from build123d import *

# Parameters (mm, degrees)
SKETCH_1_R                     = 17
EXTRUDE_1_DEPTH                = 3
SKETCH_2_R                     = 17
SKETCH_2_R_2                   = 15
EXTRUDE_2_DEPTH                = 40
SKETCH_3_R                     = 5
CUT_EXTRUDE_1_DEPTH            = 4
SKETCH_4_R                     = 17
EXTRUDE_3_DEPTH                = 7
SKETCH_5_W                     = 20.2
SKETCH_5_H                     = 20.2
EXTRUDE_4_DEPTH                = 30
HOLE_WIZARD_M5_2_D             = 5.5
HOLE_WIZARD_M5_2_CSINK_D       = 5.55
HOLE_WIZARD_M5_2_CSINK_ANGLE   = 90
HOLE_WIZARD_M2_5_2_D           = 2.9
HOLE_WIZARD_M2_5_2_DEPTH       = 3
HOLE_WIZARD_M2_5_2_CSINK_D     = 2.95
HOLE_WIZARD_M2_5_2_CSINK_ANGLE = 90
SKETCH_12_W                    = 47.187362465
SKETCH_12_H                    = 89.366632215
CUT_EXTRUDE_2_DEPTH            = 18


with BuildPart() as part:
    # 草图1 → 凸台-拉伸1 (new body)
    with BuildSketch(Plane.XY):
        Circle(SKETCH_1_R)
    extrude(amount=EXTRUDE_1_DEPTH)

    # 草图2 → 凸台-拉伸2 (add)
    with BuildSketch(Plane.XY.offset(3)):
        Circle(SKETCH_2_R)
        Circle(SKETCH_2_R_2, mode=Mode.SUBTRACT)
    extrude(amount=EXTRUDE_2_DEPTH)

    # 草图3 → 切除-拉伸1 (cut, through all)
    with BuildSketch(Plane.XY.offset(3)):
        Circle(SKETCH_3_R)
    extrude(amount=-CUT_EXTRUDE_1_DEPTH, mode=Mode.SUBTRACT)

    # 草图4 → 凸台-拉伸3 (add)
    with BuildSketch(Plane.XY.offset(43)):
        Circle(SKETCH_4_R)
        Polygon((-4.443145751, 10.1), (4.443145751, 10.1), (10.1, 4.443145751), (10.1, -4.443145751), (4.443145751, -10.1), (-4.443145751, -10.1), (-10.1, -4.443145751), (-10.1, 4.443145751), align=None, mode=Mode.SUBTRACT)
    extrude(amount=EXTRUDE_3_DEPTH)

    # 草图5 → 凸台-拉伸4 (add)
    with BuildSketch(Plane.XY.offset(50)):
        with BuildLine():
            Line((9.49684158, 14.1), (-9.49684158, 14.1))
            ThreePointArc((-9.49684158, 14.1), (-12.02081528, 12.02081528), (-14.1, 9.49684158))
            Line((-14.1, 9.49684158), (-14.1, -9.496842588))
            ThreePointArc((-14.1, -9.496842588), (-12.020815678, -12.020815678), (-9.496842588, -14.1))
            Line((-9.496842588, -14.1), (9.49684158, -14.1))
            ThreePointArc((9.49684158, -14.1), (12.02081528, -12.02081528), (14.1, -9.49684158))
            Line((14.1, -9.49684158), (14.1, 9.49684158))
            ThreePointArc((14.1, 9.49684158), (12.02081528, 12.02081528), (9.49684158, 14.1))
        make_face()
        Rectangle(SKETCH_5_W, SKETCH_5_H, mode=Mode.SUBTRACT)
    extrude(amount=EXTRUDE_4_DEPTH)

    # M5 间隙孔2 (through all)
    with Locations(Plane(origin=(0, 14.1, 0), x_dir=(1, 0, 0), z_dir=(0, 1, 0))):
        with Locations((0, -56), (0, -71)):
            CounterSinkHole(HOLE_WIZARD_M5_2_D / 2, HOLE_WIZARD_M5_2_CSINK_D / 2, counter_sink_angle=HOLE_WIZARD_M5_2_CSINK_ANGLE)

    # M2.5 间隙孔2
    with Locations(Plane.XY.offset(3)):
        with Locations((11, 0), (7.778174593, -7.778174593), (0, -11), (-7.778174593, -7.778174593), (-11, 0), (-7.778174593, 7.778174593), (0, 11), (7.778174593, 7.778174593)):
            CounterSinkHole(HOLE_WIZARD_M2_5_2_D / 2, HOLE_WIZARD_M2_5_2_CSINK_D / 2, depth=HOLE_WIZARD_M2_5_2_DEPTH, counter_sink_angle=HOLE_WIZARD_M2_5_2_CSINK_ANGLE)

    # 草图12 → 切除-拉伸2 (cut)
    with BuildSketch(Plane(origin=(0, 0, 0), x_dir=(1, 0, 0), z_dir=(0, 1, 0))):
        with Locations((-0.779036645, -41.61129095)):
            Rectangle(SKETCH_12_W, SKETCH_12_H)
    extrude(amount=-CUT_EXTRUDE_2_DEPTH, mode=Mode.SUBTRACT)


solid = part.part
Read the model definition and answer for the solid it produces. Units are mm, in the model's axes. A direction names the side the tool comes from. Round coordinates to 2 decimals unless told otherwise and drop trailing zeros. Write each loop counter-clockwise with the first axis right and the second up, starting at its lowest first coordinate (ties: lowest second). Pieces come first, ordered by that corner, then holes.
1. The part is cut by section C-C, the plane y = 11. Determine the outline of the cut face in (x, z) (3 decimals).
2. The part is cut by section A-A, the plane x = 0. Determine the outline of the cut face in (y, z) (3 decimals), then the cut area to 3 significant figures.
3. Straight lines are drawn through the part: L1, parallel to Z at x = 0, y = 11.6; L2, parallel to X at y = 5.75, z = 77; L3, parallel to Z at x = 0, y = 12.7. For each, find the intervals that lie inside material, in ascending order.
4. Determine the mould class of faces 6 (the face through (-14, 0, 48)), 7 (the face through (0, 11, 43)), 8 (the face through (-0.2, 10.3, 80)) for opening direction Z: pulls with the +Z half, pulls with the -Z half, needs draft (parallel to the pull), parting line crosses it, or undercut.
5. Given pin 1 Ø12 at (x, z) = (10, 24) entering from +Y; pin 2 Ø4.5 at (x, y) = (-2.5, 4) entering from +Z; pin 3 Ø2.5 at (x, y) = (-7.78, 7.78) entering from -Z; pin 4 Ø3.5 at (x, z) = (0, 71) entering from +Y, each flat-ended and moving along its own axis, determine where each tip first touches the part or whether it passes through.
6. The part is cut by section B-B, the plane z = 56. Determine the outline of the cut face in (x, y) (3 decimals), then the cut area to 3 significant figures.
7. Which of the six approach directions +Z, -Z, +X, -X, +Y, -Y give full straight-line access (tool end or side, diameter ignored) to faces 1 (the face through (14.1, 5, 65)), 2 (the face through (-14.1, 5, 65)), 3 (the face through (0, 14.1, 65)), 4 (the face through (-8, 8, 50)), 5 (the face through (-11.03, 1.45, 1.47))?
8. The part is cut by section D-D, the plane z = 64. Determine the outline of the cut face in (x, y), then the cut area to 3 significant figures.
Values:
1. outline: (-12.961, 0) - (-1.45, 0) - (-1.45, 2.975) - (-1.475, 3) - (-10.198, 3) - (-10.198, 43) - (10.198, 43) - (10.198, 3) - (1.475, 3) - (1.45, 2.975) - (1.45, 0) - (12.961, 0) - (12.961, 80) - (-12.961, 80) - close; hole circle Ø5.5 at (0, 56); hole circle Ø5.5 at (0, 71)
2. outline: (5, 0) - (9.55, 0) - (9.55, 2.975) - (9.525, 3) - (5, 3) - close; (10.1, 43) - (15, 43) - (15, 3) - (12.475, 3) - (12.45, 2.975) - (12.45, 0) - (17, 0) - (17, 50) - (14.1, 50) - (14.1, 53.225) - (14.075, 53.25) - (10.1, 53.25) - close; (10.1, 58.75) - (14.075, 58.75) - (14.1, 58.775) - (14.1, 68.225) - (14.075, 68.25) - (10.1, 68.25) - close; (10.1, 73.75) - (14.075, 73.75) - (14.1, 73.775) - (14.1, 80) - (10.1, 80) - close
2. area: 232 mm2
3. L1: z = 43 to 53.25, 58.75 to 68.25, 73.75 to 80
3. L2: x = -14.1 to -10.1, 10.1 to 14.1
3. L3: z = 0 to 3, 43 to 53.25, 58.75 to 68.25, 73.75 to 80
4. face 6: needs draft
4. face 7: undercut
4. face 8: pulls with the +Z half
5. pin 1: stops at y = 16.52
5. pin 2: stops at z = 3
5. pin 3: stops at z = 43
5. pin 4: passes through
6. outline: (-14.1, 0) - (-10.1, 0) - (-10.1, 10.1) - (-2.75, 10.1) - (-2.75, 14.075) - (-2.775, 14.1) - (-9.497, 14.1) arc R17 ccw to (-14.1, 9.497) - close; (2.75, 10.1) - (10.1, 10.1) - (10.1, 0) - (14.1, 0) - (14.1, 9.497) arc R17 ccw to (9.497, 14.1) - (2.775, 14.1) - (2.75, 14.075) - close
6. area: 153 mm2
7. face 1: +Z, +X, +Y, -Y
7. face 2: +Z, -X, +Y, -Y
7. face 3: +Z, +X, -X, +Y
7. face 4: +Z, -Y
7. face 5: -Z, -Y
8. outline: (-14.1, 0) - (-10.1, 0) - (-10.1, 10.1) - (10.1, 10.1) - (10.1, 0) - (14.1, 0) - (14.1, 9.5) arc R17 ccw to (9.5, 14.1) - (-9.5, 14.1) arc R17 ccw to (-14.1, 9.5) - close
8. area: 175 mm2
